from build123d import *

# Parameters (mm, degrees)
SKETCH1_R     = 7.647
BASENUT_DEPTH = 16.9


with BuildPart() as part:
    # Sketch1 → BaseNut (new body)
    with BuildSketch(Plane.XY):
        Polygon((7.794228634, -13.5), (15.588457268, 0), (7.794228634, 13.5), (-7.794228634, 13.5), (-15.588457268, 0), (-7.794228634, -13.5), align=None)
        Circle(SKETCH1_R, mode=Mode.SUBTRACT)
    extrude(amount=-BASENUT_DEPTH)

    # Sketch2 → Double-Chamfer (revolve, cut)
    with BuildSketch(Plane(origin=(0, 0, 0), x_dir=(1, 0, 0), z_dir=(0, 1, 0))):
        Polygon((-15.588457268, 16.9), (-13.125, 16.9), (-15.588457268, 15.477722283), align=None)
        Polygon((-15.588457268, 1.422277717), (-15.588457268, 0), (-13.125, 0), align=None)
    revolve(axis=Axis((0, 0, -3.375940562), (0, 0, 1)), mode=Mode.SUBTRACT)


solid = part.part
Could you check a few things on this model? Use its own coordinates, in mm. Round coordinates to 2 decimals unless told otherwise and drop trailing zeros. Order: outer loops, then holes, each group sorted by start corner. A loop starts at its lowest first (then second) coordinate and runs counter-clockwise, first axis right, second up.
(1) If we mould it in two halves opening along X, with no side actions, what happens to faces 1 (the cylindrical face through (3.5, -6.8, -8.3)), 2 (the flat face through (11.64, -6.84, -8.33)), 3 (the conical face through (2.879, 12.963, -0.089)), 4 (the flat face through (0, 13.5, -8))? For each: released by +X, released by -X, zero draft, split by the parting line, or undercut.
Response values:
face 1: undercut
face 2: released by +X
face 3: split by the parting line
face 4: zero draft
(2) I'm going to push a flat-ended pin straight in: pin 1 (2 mm diameter, centred on y = -8, z = -12, fed in from +X). Where does the tip first touch, or does it pass through?
Response values:
pin 1: stops at x = 11.55
(3) Imagine slicing it at B-B (x = 0). Write out the boundary of the cut face in (y, z) (1 decimal).
Response values:
outline: (-13.5, -16.7) - (-13.1, -16.9) - (-7.6, -16.9) - (-7.6, 0) - (-13.1, 0) - (-13.5, -0.2) - close; (7.6, -16.9) - (13.1, -16.9) - (13.5, -16.7) - (13.5, -0.2) - (13.1, 0) - (7.6, 0) - close
(4) Please list where these lines run through material, in increasing order: line 1 along Y through (x, z) = (0, -11.25); line 2 along Y through (x, z) = (5.5, -12.25); line 3 along X through (y, z) = (-4, -7.75).
Response values:
line 1: y = -13.5 to -7.65, 7.65 to 13.5
line 2: y = -13.5 to -5.31, 5.31 to 13.5
line 3: x = -13.28 to -6.52, 6.52 to 13.28
(5) Imagine slicing it at A-A (z = -5.5). Write out the boundary of the cut face in (x, y).
Response values:
outline: (-15.59, 0) - (-7.79, -13.5) - (7.79, -13.5) - (15.59, 0) - (7.79, 13.5) - (-7.79, 13.5) - close; hole circle Ø15.29 at (0, 0)
